from build123d import *

# Parameters (mm, degrees)
SKETCH2_W                                   = 151.60625
SKETCH2_H                                   = 3.175
BOSS_EXTRUDE2_DEPTH                         = 101.6
CSK_FOR_1_4_FLAT_HEAD_MACHINE_SCREW_2_COUNT = 2
CSK_FOR_1_4_FLAT_HEAD_MACHINE_SCREW_2_PITCH = 25.4
CSK_FOR_1_4_FLAT_HEAD_MACHINE_SCREW_3_COUNT = 2
CSK_FOR_1_4_FLAT_HEAD_MACHINE_SCREW_3_PITCH = 80.321852568
CSK_FOR_1_4_FLAT_HEAD_MACHINE_SCREW_4_COUNT = 2
CSK_FOR_1_4_FLAT_HEAD_MACHINE_SCREW_4_PITCH = 76.2
CUT_EXTRUDE1_DEPTH                          = 4.175
CHAMFER1_SIZE                               = 0.7874


with BuildPart() as part:
    # Sketch2 → Boss-Extrude2 (new body)
    with BuildSketch(Plane.XY):
        with Locations((75.803125, -1.5875)):
            Rectangle(SKETCH2_W, SKETCH2_H)
    extrude(amount=-BOSS_EXTRUDE2_DEPTH)

    # Sketch4 → CSK for 1/4 Flat Head Machine Screw (100)1 (revolve, cut)
    with BuildSketch(Plane(origin=(63.5, -3.175, -38.1), x_dir=(0, 0, -1), z_dir=(1, 0, 0))):
        Polygon((0, 0), (0, 3.175), (3.3782, 3.175), (3.3782, 2.568232241), (6.4389, 0), align=None)
    csk_for_1_4_flat_head_machine_screw_100 = revolve(axis=Axis((63.5, -9.525, -38.1), (0, 1, 0)), mode=Mode.SUBTRACT)

    # CSK for 1_4 Flat Head Machine Screw  2: CSK for 1/4 Flat Head Machine Screw (100)1 ×2
    with Locations(*[(0, 0, -i * CSK_FOR_1_4_FLAT_HEAD_MACHINE_SCREW_2_PITCH) for i in range(1, CSK_FOR_1_4_FLAT_HEAD_MACHINE_SCREW_2_COUNT)]):
        add(csk_for_1_4_flat_head_machine_screw_100, mode=Mode.SUBTRACT)

    # CSK for 1_4 Flat Head Machine Screw  3: CSK for 1/4 Flat Head Machine Screw (100)1 ×2
    with Locations(*[Vector(0.948683298, 0, -0.316227766) * (i * CSK_FOR_1_4_FLAT_HEAD_MACHINE_SCREW_3_PITCH) for i in range(1, CSK_FOR_1_4_FLAT_HEAD_MACHINE_SCREW_3_COUNT)]):
        add(csk_for_1_4_flat_head_machine_screw_100, mode=Mode.SUBTRACT)

    # CSK for 1_4 Flat Head Machine Screw  4: CSK for 1/4 Flat Head Machine Screw (100)1 ×2
    with Locations(*[(i * CSK_FOR_1_4_FLAT_HEAD_MACHINE_SCREW_4_PITCH, 0, 0) for i in range(1, CSK_FOR_1_4_FLAT_HEAD_MACHINE_SCREW_4_COUNT)]):
        add(csk_for_1_4_flat_head_machine_screw_100, mode=Mode.SUBTRACT)

    # Sketch5 → Cut-Extrude1 (cut, through all)
    with BuildSketch(Plane.XZ.offset(3.175)):
        with BuildLine():
            Line((3.175, 0), (0, 0))
            Line((0, 0), (0, -3.175))
            ThreePointArc((0, -3.175), (0.92993597, -0.92993597), (3.175, 0))
        make_face()
        with BuildLine():
            Line((0, -101.6), (0, -98.425))
            ThreePointArc((0, -98.425), (0.92993597, -100.67006403), (3.175, -101.6))
            Line((3.175, -101.6), (0, -101.6))
        make_face()
    extrude(amount=-CUT_EXTRUDE1_DEPTH, mode=Mode.SUBTRACT)

    # Chamfer1
    chamfer1_edges = [part.edges().sort_by_distance(p)[0] for p in [
        (77.390625, 0, -101.6),
        (77.390625, 0, 0),
        (0, 0, -50.8),
        (0.92993597, 0, -0.92993597),
        (151.60625, 0, -50.8),
        (0.92993597, 0, -100.67006403),
    ]]
    chamfer(chamfer1_edges, length=CHAMFER1_SIZE)


solid = part.part
Can you work these out from the model? Positions are in its coordinate system, mm. Give positions to 0.01 mm unless a question says otherwise; leave off trailing zeros. Loops run counter-clockwise (first coordinate to the right, second up) from the corner with the lowest first, then second, coordinate; pieces in that order, holes last. Notation, with made-up numbers: (61.5, 35) -> (93.5, 35) arc R36 cw to (93.5, 69) -> close; hole circle Ø11 at (7, 75.5). An arc over 180 degrees is marked (long way). Write item = value, one per line.
1) Suppose I cut it at C-C on y = -1.55. Write out the boundary of the cut face in (x, z) (3 decimals).
Check result:
outline = (0, -98.425) arc R3.175 ccw to (3.175, -101.6) -> (151.606, -101.6) -> (151.606, 0) -> (3.175, 0) arc R3.175 ccw to (0, -3.175) -> close; hole circle Ø9.005 at (63.5, -63.5); hole circle Ø9.005 at (63.5, -38.1); hole circle Ø9.005 at (139.7, -63.5); hole circle Ø9.005 at (139.7, -38.1)
2) I need wall thicknesses on L1, parallel to Z at x = 63.5, y = -0.15; L2, parallel to Z at x = 63.5, y = -0.25; L3, parallel to X at y = -0.4, z = -63.5. Which ranges of each line are inside material? Lowest first, please. Write a range as from..to.
Check result:
L1 = -100.96..-66.88, -60.12..-41.48, -34.72..-0.64
L2 = -101.06..-66.88, -60.12..-41.48, -34.72..-0.54
L3 = 0.39..60.12, 66.88..136.32, 143.08..151.22
3) Thinking about a two-plate mould opening in X: for faces 1 (the flat face through (75, -3.175, -50)), 2 (the conical face through (136.69, -0.77, -40.02)), 3 (the conical face through (1.31, -0.22, -100.25)), which applies, released by +X, released by -X, zero draft, split by the parting line, or undercut?
Check result:
face_1 = zero draft
face_2 = undercut
face_3 = released by -X
4) Suppose I cut it at A-A on x = 139.7. Write out the boundary of the cut face in (y, z) (3 decimals).
Check result:
outline = (-3.175, -101.6) -> (-0.787, -101.6) -> (0, -100.813) -> (0, -66.878) -> (-0.607, -66.878) -> (-3.175, -69.939) -> close; (-3.175, -57.061) -> (-0.607, -60.122) -> (0, -60.122) -> (0, -41.478) -> (-0.607, -41.478) -> (-3.175, -44.539) -> close; (-3.175, -31.661) -> (-0.607, -34.722) -> (0, -34.722) -> (0, -0.787) -> (-0.787, 0) -> (-3.175, 0) -> close
5) Suppose I cut it at B-B on z = -63.5. Write out the boundary of the cut face in (x, y) (3 decimals).
Check result:
outline = (0, -3.175) -> (57.061, -3.175) -> (60.122, -0.607) -> (60.122, 0) -> (0.787, 0) -> (0, -0.787) -> close; (66.878, -0.607) -> (69.939, -3.175) -> (133.261, -3.175) -> (136.322, -0.607) -> (136.322, 0) -> (66.878, 0) -> close; (143.078, -0.607) -> (146.139, -3.175) -> (151.606, -3.175) -> (151.606, -0.787) -> (150.819, 0) -> (143.078, 0) -> close
6) Will these pins go through, and if not, where does the flat tip stop? pin 1 (9 mm diameter, centred on x = 63.5, z = -38.1, fed in from -Y); pin 2 (11 mm diameter, centred on x = 139.7, z = -38.1, fed in from -Y).
Check result:
pin_1 = -1.55
pin_2 = -2.39
